Job drawing, mm, ordinate dimensions from the low corner. One solid piece. A direction names the side the tool comes from. Give positions to 0.01 mm unless a question says otherwise; leave off trailing zeros. Loops run counter-clockwise (first coordinate to the right, second up) from the corner with the lowest first, then second, coordinate; pieces in that order, holes last. Notation, with made-up numbers: M 56.5,71 L 104.5,71 A23 cw 104.5,99 Z; hole C 32.5,-0.75 d9. An arc over 180 degrees is marked long. Answer in a Markdown table with one row per item.
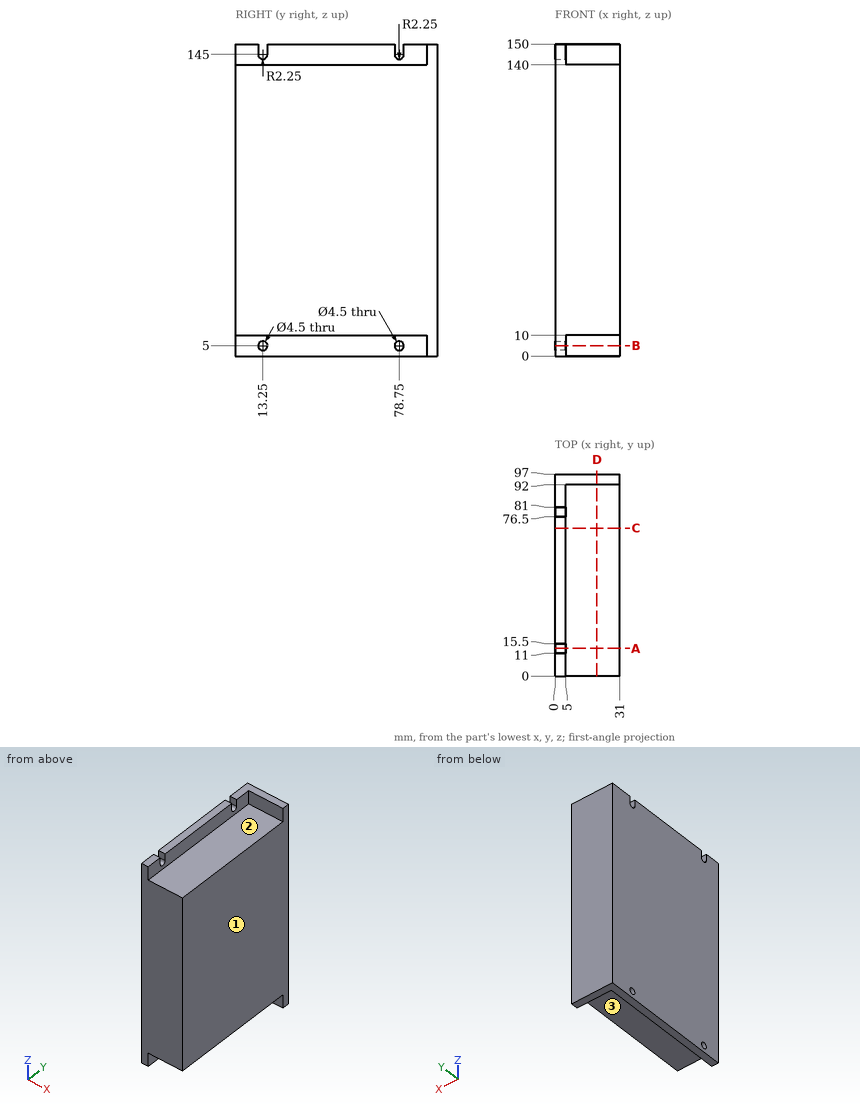
(1) Saw through at C-C (y = 71). Write the cut outline in (x, z), plus the area to 3 significant figures.
Recorded:
| item | result |
|---|---|
| outline | M 0,0 L 5,0 L 5,10 L 31,10 L 31,140 L 5,140 L 5,150 L 0,150 Z |
| area | 4,130 mm^2 |
(2) Saw through at D-D (x = 20). Write the cut outline in (y, z).
Recorded:
| item | result |
|---|---|
| outline | M 0,10 L 92,10 L 92,0 L 97,0 L 97,150 L 92,150 L 92,140 L 0,140 Z |
(3) Drill centre lines: line 1 along Y through (x, z) = (2, 5); line 2 along Z through (x, y) = (2, 13); line 3 along Z through (x, y) = (7.5, 74.5). Where is each one in solid material? Low to high.
Recorded:
| item | result |
|---|---|
| line 1 | y = 0 to 11, 15.5 to 76.5, 81 to 97 |
| line 2 | z = 0 to 2.76, 7.24 to 142.76 |
| line 3 | z = 10 to 140 |
(4) Saw through at A-A (y = 13.25). Write the cut outline in (x, z), plus the area to 3 significant figures.
Recorded:
| item | result |
|---|---|
| outline | M 0,0 L 5,0 L 5,2.75 L 0,2.75 Z; M 0,7.25 L 5,7.25 L 5,10 L 31,10 L 31,140 L 5,140 L 5,142.75 L 0,142.75 Z |
| area | 4,070 mm^2 |
(5) Which spindle directions (+Z, -Z, +X, -X, +Y, -Y) get a long thin tool onto all of the face, cutting with end or side? Do the marked faces 1, 2 and 3. Say none if no direction does.
Recorded:
| item | result |
|---|---|
| face 1 | +Z, -Z, +X, +Y, -Y |
| face 2 | +Z, +X, -Y |
| face 3 | -Z, +X, -Y |
(6) Pin check, flat tips, straight feed: pin 1 Ø6 at (x, y) = (27, 15.5) entering from +Z; pin 2 Ø8 at (y, z) = (58, 4.5) entering from +X; pin 3 Ø5 at (x, y) = (8.5, 69.5) entering from -Z. Stop position of each tip, or through.
Recorded:
| item | result |
|---|---|
| pin 1 | stops at z = 140 |
| pin 2 | stops at x = 5 |
| pin 3 | stops at z = 10 |
(7) Saw through at B-B (z = 5). Write the cut outline in (x, y).
Recorded:
| item | result |
|---|---|
| outline | M 0,0 L 5,0 L 5,11 L 0,11 Z; M 0,15.5 L 5,15.5 L 5,76.5 L 0,76.5 Z; M 0,81 L 5,81 L 5,92 L 31,92 L 31,97 L 0,97 Z |
